The model under review builds one solid part; all positions refer to its coordinate system, in mm. A direction names the side the tool comes from. Give positions to 0.01 mm unless a question says otherwise; leave off trailing zeros. Write each loop counter-clockwise with the first axis right and the second up, starting at its lowest first coordinate (ties: lowest second). Pieces come first, ordered by that corner, then holes. Notation, with made-up numbers: (8.25, -35.5) - (56.25, -35.5) arc R19 ccw to (56.25, -30.5) - close; hole circle Ø11 at (48, -21). An arc over 180 degrees is marked (long way). Write item = value, one per line.
```python
from build123d import *

# Parameters (mm, degrees)
SKETCH1_W           = 169.3418
SKETCH1_H           = 254
BOSS_EXTRUDE1_DEPTH = 45.72
SKETCH2_W           = 149.0218
SKETCH2_H           = 233.68
CUT_EXTRUDE1_DEPTH  = 40.64
CUT_EXTRUDE10_REACH = 310.679
F_12_PIN_MOUNT_R    = 2.7999944
CUT_EXTRUDE3_DEPTH  = 5.499989
CUT_EXTRUDE5_REACH  = 310.679
CUT_EXTRUDE6_START  = -254
CUT_EXTRUDE6_DEPTH  = 10.16
SKETCH6_R           = 2.7999944
CUT_EXTRUDE7_DEPTH  = 5.499989
CUT_EXTRUDE8_START  = -248.500011
SKETCH6_2_R         = 2.7999944
CUT_EXTRUDE8_DEPTH  = 5.499989
SKETCH7_R           = 5
BOSS_EXTRUDE2_DEPTH = 6.35
CUT_EXTRUDE9_START  = 6.35
SKETCH8_R           = 2.7999944
CUT_EXTRUDE9_DEPTH  = 5.499989


with BuildPart() as part:
    # Sketch1 → Boss-Extrude1 (new body)
    with BuildSketch(Plane(origin=(0, 0, 0), x_dir=(1, 0, 0), z_dir=(0, 1, 0))):
        with Locations((84.6709, 127)):
            Rectangle(SKETCH1_W, SKETCH1_H)
    extrude(amount=BOSS_EXTRUDE1_DEPTH)

    # Sketch2 → Cut-Extrude1 (cut)
    with BuildSketch(Plane(origin=(0, 45.72, 0), x_dir=(1, 0, 0), z_dir=(0, 1, 0))):
        with Locations((84.6709, 127)):
            Rectangle(SKETCH2_W, SKETCH2_H)
    extrude(amount=-CUT_EXTRUDE1_DEPTH, mode=Mode.SUBTRACT)

    # Cut-Sweep2: sweep along a path in Sketch3
    with BuildLine(Plane(origin=(0, 45.72, 0), x_dir=(1, 0, 0), z_dir=(0, 1, 0))) as cut_sweep2_path:
        Line((6.35, 11.43), (6.35, 242.57))
        ThreePointArc((6.35, 242.57), (7.837897552, 246.162102448), (11.43, 247.65))
        Line((11.43, 247.65), (157.9118, 247.65))
        ThreePointArc((157.9118, 247.65), (161.503902448, 246.162102448), (162.9918, 242.57))
        Line((162.9918, 242.57), (162.9918, 11.43))
        ThreePointArc((162.9918, 11.43), (161.503902448, 7.837897552), (157.9118, 6.35))
        Line((157.9118, 6.35), (11.43, 6.35))
        ThreePointArc((11.43, 6.35), (7.837897552, 7.837897552), (6.35, 11.43))
    # Sketch4 → Cut-Sweep2 (sweep, cut)
    with BuildSketch(Plane.XY.offset(-15.24)):
        Polygon((4.064, 45.72), (3.272383398, 43.942), (7.141616602, 43.942), (6.35, 45.72), align=None)
    sweep(path=cut_sweep2_path.line, mode=Mode.SUBTRACT)

    # Sketch13 → Cut-Extrude10 (cut, up to next)
    with BuildSketch(Plane(origin=(169.3418, 0, 0), x_dir=(0, 0, -1), z_dir=(1, 0, 0)), mode=Mode.PRIVATE) as cut_extrude10_sk1:
        with BuildLine():
            Line((37.955714122, 28.956), (36.5125, 28.956))
            ThreePointArc((36.5125, 28.956), (35.434869265, 28.509630735), (34.9885, 27.432))
            Line((34.9885, 27.432), (34.9885, 16.764))
            ThreePointArc((34.9885, 16.764), (35.434869265, 15.686369265), (36.5125, 15.24))
            Line((36.5125, 15.24), (37.955714122, 15.24))
            ThreePointArc((37.955714122, 15.24), (38.329218307, 15.142182673), (38.606829629, 14.873844156))
            ThreePointArc((38.606829629, 14.873844156), (41.179361214, 12.387240562), (44.6405, 11.4808))
            Line((44.6405, 11.4808), (66.3575, 11.4808))
            ThreePointArc((66.3575, 11.4808), (69.314150798, 12.129608753), (71.727465925, 13.956805195))
            ThreePointArc((71.727465925, 13.956805195), (71.987895615, 14.153984667), (72.306958651, 14.224))
            Line((72.306958651, 14.224), (74.4855, 14.224))
            ThreePointArc((74.4855, 14.224), (75.563130735, 14.670369265), (76.0095, 15.748))
            Line((76.0095, 15.748), (76.0095, 28.448))
            ThreePointArc((76.0095, 28.448), (75.563130735, 29.525630735), (74.4855, 29.972))
            Line((74.4855, 29.972), (72.306958651, 29.972))
            ThreePointArc((72.306958651, 29.972), (71.987895615, 30.042015333), (71.727465925, 30.239194805))
            ThreePointArc((71.727465925, 30.239194805), (69.314150798, 32.066391247), (66.3575, 32.7152))
            Line((66.3575, 32.7152), (44.6405, 32.7152))
            ThreePointArc((44.6405, 32.7152), (41.179361214, 31.808759438), (38.606829629, 29.322155844))
            ThreePointArc((38.606829629, 29.322155844), (38.329218307, 29.053817327), (37.955714122, 28.956))
        make_face()
    cut_extrude10_tool1 = extrude(cut_extrude10_sk1.sketch, amount=-CUT_EXTRUDE10_REACH, mode=Mode.PRIVATE) & part.part
    # Sketch13 → Cut-Extrude10 (cut, up to next)
    with BuildSketch(Plane(origin=(169.3418, 0, 0), x_dir=(0, 0, -1), z_dir=(1, 0, 0)), mode=Mode.PRIVATE) as cut_extrude10_sk2:
        with BuildLine():
            Line((180.957714122, 28.956), (179.5145, 28.956))
            ThreePointArc((179.5145, 28.956), (178.436869265, 28.509630735), (177.9905, 27.432))
            Line((177.9905, 27.432), (177.9905, 16.764))
            ThreePointArc((177.9905, 16.764), (178.436869265, 15.686369265), (179.5145, 15.24))
            Line((179.5145, 15.24), (180.957714122, 15.24))
            ThreePointArc((180.957714122, 15.24), (181.331218307, 15.142182673), (181.608829629, 14.873844156))
            ThreePointArc((181.608829629, 14.873844156), (184.181361214, 12.387240562), (187.6425, 11.4808))
            Line((187.6425, 11.4808), (209.3595, 11.4808))
            ThreePointArc((209.3595, 11.4808), (212.316150798, 12.129608753), (214.729465925, 13.956805195))
            ThreePointArc((214.729465925, 13.956805195), (214.989895615, 14.153984667), (215.308958651, 14.224))
            Line((215.308958651, 14.224), (217.4875, 14.224))
            ThreePointArc((217.4875, 14.224), (218.565130735, 14.670369265), (219.0115, 15.748))
            Line((219.0115, 15.748), (219.0115, 28.448))
            ThreePointArc((219.0115, 28.448), (218.565130735, 29.525630735), (217.4875, 29.972))
            Line((217.4875, 29.972), (215.308958651, 29.972))
            ThreePointArc((215.308958651, 29.972), (214.989895615, 30.042015333), (214.729465925, 30.239194805))
            ThreePointArc((214.729465925, 30.239194805), (212.316150798, 32.066391247), (209.3595, 32.7152))
            Line((209.3595, 32.7152), (187.6425, 32.7152))
            ThreePointArc((187.6425, 32.7152), (184.181361214, 31.808759438), (181.608829629, 29.322155844))
            ThreePointArc((181.608829629, 29.322155844), (181.331218307, 29.053817327), (180.957714122, 28.956))
        make_face()
    cut_extrude10_tool2 = extrude(cut_extrude10_sk2.sketch, amount=-CUT_EXTRUDE10_REACH, mode=Mode.PRIVATE) & part.part
    add(cut_extrude10_tool1.solids().sort_by_distance((169.3418, 22.098, -55.674803))[0], mode=Mode.SUBTRACT)
    add(cut_extrude10_tool2.solids().sort_by_distance((169.3418, 22.098, -198.676803))[0], mode=Mode.SUBTRACT)

    # 12 pin mount → Cut-Extrude3 (cut)
    with BuildSketch(Plane(origin=(169.3418, 0, 0), x_dir=(0, 0, -1), z_dir=(1, 0, 0))):
        with Locations((77.978, 34.036)):
            Circle(F_12_PIN_MOUNT_R)
        with Locations((77.978, 10.16)):
            Circle(F_12_PIN_MOUNT_R)
        with Locations((33.02, 10.16)):
            Circle(F_12_PIN_MOUNT_R)
        with Locations((33.02, 34.036)):
            Circle(F_12_PIN_MOUNT_R)
        with Locations((176.022, 34.036)):
            Circle(F_12_PIN_MOUNT_R)
        with Locations((220.98, 34.036)):
            Circle(F_12_PIN_MOUNT_R)
        with Locations((220.98, 10.16)):
            Circle(F_12_PIN_MOUNT_R)
        with Locations((176.022, 10.16)):
            Circle(F_12_PIN_MOUNT_R)
    extrude(amount=-CUT_EXTRUDE3_DEPTH, mode=Mode.SUBTRACT)

    # 4 pin connector → Cut-Extrude5 (cut, up to next)
    with BuildSketch(Plane.XY, mode=Mode.PRIVATE) as cut_extrude5_sk1:
        with BuildLine():
            Line((32.6263, 31.877), (47.1043, 31.877))
            ThreePointArc((47.1043, 31.877), (49.798376836, 30.761076836), (50.9143, 28.067))
            Line((50.9143, 28.067), (50.9143, 14.7066))
            ThreePointArc((50.9143, 14.7066), (49.798376836, 12.012523164), (47.1043, 10.8966))
            Line((47.1043, 10.8966), (32.6263, 10.8966))
            ThreePointArc((32.6263, 10.8966), (29.932223164, 12.012523164), (28.8163, 14.7066))
            Line((28.8163, 14.7066), (28.8163, 28.067))
            ThreePointArc((28.8163, 28.067), (29.932223164, 30.761076836), (32.6263, 31.877))
        make_face()
    cut_extrude5_tool1 = extrude(cut_extrude5_sk1.sketch, amount=-CUT_EXTRUDE5_REACH, mode=Mode.PRIVATE) & part.part
    add(cut_extrude5_tool1.solids().sort_by_distance((39.8653, 21.3868, 0))[0], mode=Mode.SUBTRACT)

    # Sketch5<2> → Cut-Extrude6 (cut)
    with BuildSketch(Plane.XY.offset(CUT_EXTRUDE6_START)):
        with BuildLine():
            Line((32.6263, 31.877), (47.1043, 31.877))
            ThreePointArc((47.1043, 31.877), (49.798376836, 30.761076836), (50.9143, 28.067))
            Line((50.9143, 28.067), (50.9143, 14.7066))
            ThreePointArc((50.9143, 14.7066), (49.798376836, 12.012523164), (47.1043, 10.8966))
            Line((47.1043, 10.8966), (32.6263, 10.8966))
            ThreePointArc((32.6263, 10.8966), (29.932223164, 12.012523164), (28.8163, 14.7066))
            Line((28.8163, 14.7066), (28.8163, 28.067))
            ThreePointArc((28.8163, 28.067), (29.932223164, 30.761076836), (32.6263, 31.877))
        make_face()
    extrude(amount=CUT_EXTRUDE6_DEPTH, mode=Mode.SUBTRACT)

    # Sketch6 → Cut-Extrude7 (cut)
    with BuildSketch(Plane.XY):
        with Locations((55.0418, 32.6136)):
            Circle(SKETCH6_R)
        with Locations((55.0418, 10.16)):
            Circle(SKETCH6_R)
        with Locations((24.6888, 10.16)):
            Circle(SKETCH6_R)
        with Locations((24.6888, 32.6136)):
            Circle(SKETCH6_R)
    extrude(amount=-CUT_EXTRUDE7_DEPTH, mode=Mode.SUBTRACT)

    # Sketch6<2> → Cut-Extrude8 (cut)
    with BuildSketch(Plane.XY.offset(CUT_EXTRUDE8_START)):
        with Locations((55.0418, 32.6136)):
            Circle(SKETCH6_2_R)
        with Locations((55.0418, 10.16)):
            Circle(SKETCH6_2_R)
        with Locations((24.6888, 10.16)):
            Circle(SKETCH6_2_R)
        with Locations((24.6888, 32.6136)):
            Circle(SKETCH6_2_R)
    extrude(amount=-CUT_EXTRUDE8_DEPTH, mode=Mode.SUBTRACT)

    # Sketch7 → Boss-Extrude2 (add)
    with BuildSketch(Plane(origin=(0, 5.08, 0), x_dir=(1, 0, 0), z_dir=(0, 1, 0))):
        with Locations(Location((55.4218, 82.485, 0), (0, 0, 90))):
            Circle(SKETCH7_R)
        with Locations(Location((121.0818, 82.485, 0), (0, 0, 90))):
            Circle(SKETCH7_R)
        with Locations(Location((121.0818, 171.515, 0), (0, 0, 90))):
            Circle(SKETCH7_R)
        with Locations(Location((55.4218, 171.515, 0), (0, 0, 90))):
            Circle(SKETCH7_R)
    extrude(amount=BOSS_EXTRUDE2_DEPTH)

    # Sketch8 → Cut-Extrude9 (cut)
    with BuildSketch(Plane(origin=(0, 5.08, 0), x_dir=(1, 0, 0), z_dir=(0, 1, 0)).offset(CUT_EXTRUDE9_START)):
        with Locations(Location((55.4218, 171.515, 0), (0, 0, 270))):
            Circle(SKETCH8_R)
        with Locations(Location((121.0818, 171.515, 0), (0, 0, 270))):
            Circle(SKETCH8_R)
        with Locations(Location((121.0818, 82.485, 0), (0, 0, 270))):
            Circle(SKETCH8_R)
        with Locations(Location((55.4218, 82.485, 0), (0, 0, 270))):
            Circle(SKETCH8_R)
    extrude(amount=-CUT_EXTRUDE9_DEPTH, mode=Mode.SUBTRACT)


solid = part.part
```
1. Machinability: for faces 4 (the flat face through (10.16, 26, -125)), 5 (the flat face through (164, 22, -76.01)), 6 (the conical face through (161.13, 44.65, -245.86)), 7 (the cylindrical face through (57.712, 11.001, -251.212)), which of the approach directions +Z, -Z, +X, -X, +Y, -Y give a long, thin tool a straight path to every point of the face, cutting with its end or side? Answer none if there is none.
Findings below:
face_4 = +Y
face_5 = +X
face_6 = none
face_7 = -Z
2. Insertion check: P1, Ø8, axis at x = 163.5, z = -53, coming from the +Y side; P2, Ø6, axis at y = 26, z = -40, coming from the +X side; P3, Ø5, axis at x = 120, z = -170.5, coming from the +Y side; P4, Ø1.7, axis at x = 57, z = -171, coming from the +Y side. Each pin has a flat end and moves straight along its axis. Give the tip position at first contact, or say it passes through.
Findings below:
P1 = 45.72
P2 = 10.16
P3 = 11.43
P4 = 5.93
3. Take a section at A-A on z = -52.5. Give the boundary of the cut face in (x, y), and give its area (3 significant figures).
Findings below:
outline = (0, 0) - (169.34, 0) - (169.34, 11.48) - (159.18, 11.48) - (159.18, 5.08) - (10.16, 5.08) - (10.16, 45.72) - (6.35, 45.72) - (7.14, 43.94) - (3.27, 43.94) - (4.06, 45.72) - (0, 45.72) - close; (159.18, 32.72) - (169.34, 32.72) - (169.34, 45.72) - (165.28, 45.72) - (166.07, 43.94) - (162.2, 43.94) - (162.99, 45.72) - (159.18, 45.72) - close
area = 1,460 mm²
4. For line 1 (Z direction, x = 167, y = 10); line 2 (Z direction, x = 112, y = 9.5); line 3 (X direction, y = 40.5, z = -98.5), list the stretches that pass through material, from the lowest coordinate up. Write a range as from..to.
Findings below:
line_1 = -254..-223.78, -218.18..-178.82, -173.23..-80.77, -75.18..-35.82, -30.22..0
line_2 = -254..-243.84, -10.16..0
line_3 = 0..10.16, 159.18..169.34
5. Draft analysis for pull direction X (two halves, no side actions). For faces 1 (the flat face through (55, 5.93, -172)), 2 (the flat face through (0, 23, -125)), 3 (the cylindrical face through (166.63, 34.88, -178.69)), state which applies: +X half, -X half, draft (parallel to the pull), parting line (faces both ways), or undercut.
Findings below:
face_1 = undercut
face_2 = -X half
face_3 = draft
6. Take a section at B-B on x = 66. Give the boundary of the cut face in (y, z), and give its area (3 significant figures).
Findings below:
outline = (0, -254) - (45.72, -254) - (45.72, -249.94) - (43.94, -250.73) - (43.94, -246.86) - (45.72, -247.65) - (45.72, -243.84) - (5.08, -243.84) - (5.08, -10.16) - (45.72, -10.16) - (45.72, -6.35) - (43.94, -7.14) - (43.94, -3.27) - (45.72, -4.06) - (45.72, 0) - (0, 0) - close
area = 2,110 mm²
7. Take a section at C-C on z = -114. Give the boundary of the cut face in (x, y), and give its area (3 significant figures).
Findings below:
outline = (0, 0) - (169.34, 0) - (169.34, 45.72) - (165.28, 45.72) - (166.07, 43.94) - (162.2, 43.94) - (162.99, 45.72) - (159.18, 45.72) - (159.18, 5.08) - (10.16, 5.08) - (10.16, 45.72) - (6.35, 45.72) - (7.14, 43.94) - (3.27, 43.94) - (4.06, 45.72) - (0, 45.72) - close
area = 1,680 mm²
